Geometry check sheet. Reference: the model listing, model coordinates, mm. A direction names the side the tool comes from. Round coordinates to 2 decimals unless told otherwise and drop trailing zeros. Loops run counter-clockwise (first coordinate to the right, second up) from the corner with the lowest first, then second, coordinate; pieces in that order, holes last. Notation, with made-up numbers: M 74.5,19 L 128.5,19 A28 cw 128.5,54 Z; hole C 67,-1.75 d1. An arc over 180 degrees is marked long. Answer in a Markdown table with one row per item. Add a question column.
```python
from build123d import *

# Parameters (mm, degrees)
BOX_W           = 34.5
BOX_H           = 16
BOX_DEPTH       = 59
SKETCH_R        = 4
POCKET_DEPTH    = 34.501
POCKET001_DEPTH = 3.5000000001
BOX001_W        = 45
BOX001_H        = 9.5
BOX001_DEPTH    = 50
SKETCH008_R     = 1.75
POCKET002_DEPTH = 9.5010000001
PAD_DEPTH       = 8
PAD001_DEPTH    = 2
SKETCH009_R     = 3.5
POCKET003_DEPTH = 2
PAD002_DEPTH    = 50
SKETCH013_R     = 6
PAD003_DEPTH    = 17
SKETCH019_W     = 9
SKETCH019_H     = 5.5
PAD004_DEPTH    = 2
SKETCH015_W     = 3
SKETCH015_H     = 4
GROOVE_ANGLE    = 40
SKETCH016_W     = 3
SKETCH016_H     = 4
POCKET004_DEPTH = 5
SKETCH020_W     = 6.4
SKETCH020_H     = 3
PAD005_DEPTH    = 8
SKETCH021_R     = 1.7
POCKET005_DEPTH = 13
POCKET006_DEPTH = 15
SKETCH023_W     = 34.5
SKETCH023_H     = 2
POCKET007_DEPTH = 100


with BuildPart() as pocket001:
    # Box → Box (new body)
    with BuildSketch(Plane(origin=(-18, -8, -30), x_dir=(1, 0, 0), z_dir=(0, 0, 1))):
        with Locations((17.25, 8)):
            Rectangle(BOX_W, BOX_H)
    extrude(amount=BOX_DEPTH)

    # Sketch → Pocket (cut, through all)
    with BuildSketch(Plane(origin=(16.5, -8, -30), x_dir=(0, 1, 0), z_dir=(1, 0, 0))):
        with Locations((8, 51)):
            Circle(SKETCH_R)
        with Locations((8, 6)):
            Circle(SKETCH_R)
        with BuildLine():
            ThreePointArc((12.5, 39.4999793754), (8.0000103123, 44), (3.5, 39.5))
            Line((3.5, 39.5), (3.5, 14.5))
            Line((3.5, 14.5), (6, 12))
            Line((6, 12), (10, 12))
            Line((10, 12), (12.5, 14.5))
            Line((12.5, 14.5), (12.5, 39.4999793754))
        make_face()
    extrude(amount=-POCKET_DEPTH, mode=Mode.SUBTRACT)

    # Sketch007 → Pocket001 (cut)
    with BuildSketch(Plane(origin=(-18, 8, -30), x_dir=(-1, 0, 0), z_dir=(0, 1, 0))):
        Polygon((-34.5, 39.4999793754), (-24.8503628945, 27.9999896877), (-24.8503628945, 25.9999896877), (-34.5, 14.5), align=None)
    extrude(amount=-POCKET001_DEPTH, mode=Mode.SUBTRACT)


with BuildPart() as pocket007:
    # Box001 → Box001 (new body)
    with BuildSketch(Plane(origin=(16, -14, -30), x_dir=(1, 0, 0), z_dir=(0, 0, 1))):
        with Locations((22.5, 4.75)):
            Rectangle(BOX001_W, BOX001_H)
    extrude(amount=BOX001_DEPTH)

    # Sketch008 → Pocket002 (cut, through all)
    with BuildSketch(Plane(origin=(16, -14, -30), x_dir=(1, 0, 0), z_dir=(0, -1, 0))):
        with Locations((7, 44.5)):
            Circle(SKETCH008_R)
        with Locations((7, 13.5)):
            Circle(SKETCH008_R)
        with Locations((38, 13.5)):
            Circle(SKETCH008_R)
        Polygon((14, 50), (14, 43), (8.5, 37.5), (8.5, 21.5), (14, 16), (32.692131, 16), (32.692131, 18), (45, 18), (45, 50), align=None)
        Polygon((45, 9.1923881554), (35.8076118446, 0), (45, 0), align=None)
    extrude(amount=-POCKET002_DEPTH, mode=Mode.SUBTRACT)

    # Fusion: union Pocket001
    add(pocket001.part)

    # Sketch010 → Pad (new body)
    with BuildSketch(Plane(origin=(0, 0, -30), x_dir=(1, 0, 0), z_dir=(0, 0, -1))):
        with BuildLine():
            ThreePointArc((25.4999662688, 4.4999999999), (19.1360389694, 1.8639610307), (16.5000000001, -4.4999662687))
            Line((16.5000000001, -4.4999662687), (16.5000000001, 4.4999999999))
            Line((16.5000000001, 4.4999999999), (25.4999662688, 4.4999999999))
        make_face()
    extrude(amount=-PAD_DEPTH)

    # Sketch011 → Pad001 (new body)
    with BuildSketch(Plane.YZ.offset(16.5)):
        with BuildLine():
            ThreePointArc((-3.4641016151, -22), (0, -28), (3.4641016151, -22))
            Line((-3.4641016151, -22), (3.4641016151, -22))
        make_face()
    extrude(amount=-PAD001_DEPTH)

    # Sketch009 → Pocket003 (cut)
    with BuildSketch(Plane(origin=(0, -4.5, 0), x_dir=(-1, 0, 0), z_dir=(0, 1, 0))):
        with Locations((-23, 14.5)):
            Circle(SKETCH009_R)
        with Locations((-54, -16.5)):
            Circle(SKETCH009_R)
        with Locations((-23, -16.5)):
            Circle(SKETCH009_R)
    extrude(amount=-POCKET003_DEPTH, mode=Mode.SUBTRACT)

    # Sketch012 → Pad002 (new body)
    with BuildSketch(Plane(origin=(0, 0, -30), x_dir=(1, 0, 0), z_dir=(0, 0, -1))):
        with BuildLine():
            ThreePointArc((15.9999999999, 18.0000351724), (15.4138656704, 20.9466786767), (13.7447222151, 23.4447222151))
            Line((13.7447222151, 23.4447222151), (12.6133513652, 22.3133513652))
            ThreePointArc((11.6013945082, 23.1294048681), (4.4708258711, 13.2515870556), (12.6133513652, 22.3133513652))
            Line((11.6013945082, 23.1294048681), (12.4673340514, 24.4748225384))
            ThreePointArc((12.4673340514, 24.4748225384), (4.6120940547, 24.759389746), (0.6000000001, 18.0000351024))
            Line((0.6000000001, 18.0000351024), (0.6000000001, 8))
            Line((0.6000000001, 8), (15.9999999999, 8))
            Line((15.9999999999, 18.0000351724), (15.9999999999, 8))
        make_face()
    extrude(amount=-PAD002_DEPTH)

    # Sketch013 → Pad003 (new body)
    with BuildSketch(Plane(origin=(0, 0, -30), x_dir=(1, 0, 0), z_dir=(0, 0, -1))):
        with BuildLine():
            ThreePointArc((1.3480393737, 25.435516441), (-17.5103595019, 26.8672185857), (-16.2, 8))
            Line((-16.2, 8), (0.6000000001, 8))
            Line((0.6000000001, 8), (0.6, 18.0000060082))
            ThreePointArc((4.5689954494, 24.7356963295), (1.6660458786, 21.9090475457), (0.6, 18.0000060082))
            ThreePointArc((1.3480393737, 25.435516441), (2.8268537634, 24.4796180457), (4.5689954493, 24.7356963295))
        make_face()
        with Locations((-8.7, 18)):
            Circle(SKETCH013_R, mode=Mode.SUBTRACT)
    extrude(amount=-PAD003_DEPTH)

    # Sketch019 → Pad004 (new body)
    with BuildSketch(Plane.YZ.offset(16.5)):
        with Locations((0, 19.25)):
            Rectangle(SKETCH019_W, SKETCH019_H)
    extrude(amount=-PAD004_DEPTH)

    # Sketch015 → Groove (revolve, cut)
    with BuildSketch(Plane.XZ.offset(14)):
        with Locations((17.5, 5.5)):
            Rectangle(SKETCH015_W, SKETCH015_H)
    revolve(axis=Axis((0, -14, 0), (0, 0, 1)), revolution_arc=GROOVE_ANGLE, mode=Mode.SUBTRACT)

    # Sketch016 → Pocket004 (cut)
    with BuildSketch(Plane.XZ.offset(8)):
        with Locations((-0.8999999999, 5.5)):
            Rectangle(SKETCH016_W, SKETCH016_H)
    extrude(amount=-POCKET004_DEPTH, mode=Mode.SUBTRACT)

    # Sketch020 → Pad005 (new body)
    with BuildSketch(Plane(origin=(0, 0, -30), x_dir=(1, 0, 0), z_dir=(0, 0, -1))):
        Polygon((-19.3039162536, 24.6186826549), (-12.2, 36), (-5.2, 36), (1.3480393737, 25.435516441), align=None)
        with Locations((-8.7, 32)):
            Rectangle(SKETCH020_W, SKETCH020_H, mode=Mode.SUBTRACT)
    extrude(amount=-PAD005_DEPTH)

    # Sketch021 → Pocket005 (cut)
    with BuildSketch(Plane.XZ.offset(36)):
        with Locations((-8.7, -26)):
            Circle(SKETCH021_R)
    extrude(amount=-POCKET005_DEPTH, mode=Mode.SUBTRACT)

    # Sketch022 → Pocket006 (cut, symmetric)
    with BuildSketch(Plane.XY.offset(-13)):
        Polygon((-3.7636551984, -26.55), (1.1726896031, -18), (-3.7636551984, -9.45), (-13.6363448016, -9.45), (-18.5726896031, -18), (-13.6363448016, -26.55), align=None)
    extrude(amount=POCKET006_DEPTH, both=True, mode=Mode.SUBTRACT)

    # Sketch023 → Pocket007 (cut)
    with BuildSketch(Plane.XY.offset(29)):
        with Locations((-0.75, 7)):
            Rectangle(SKETCH023_W, SKETCH023_H)
    extrude(amount=-POCKET007_DEPTH, mode=Mode.SUBTRACT)


solid = pocket007.part
```
1) Go/stop test with flat-tipped pins: pin 1 (5 mm diameter, centred on x = 15, y = -9, fed in from +Z); pin 2 (15.5 mm diameter, centred on x = -8.7, y = -18, fed in from +Z); pin 3 (1 mm diameter, centred on y = -6, z = 5.5, fed in from +X); pin 4 (10.5 mm diameter, centred on y = -9.5, z = 3.5, fed in from +X). Record where each tip stops, or that it passes through.
2) Draft check along Y on faces 5 (the cylindrical face through (-0.509, -0.521, -20.034)), 6 (the flat face through (39, -9, -14)), 7 (the flat face through (33, -14, -16)). Enter one of: +Y half, -Y half, draft (parallel to the pull), parting line (faces both ways), or undercut.
3) Cross-section at B-B, the plane x = 23. Record the boundary of the cut face in (y, z), plus the area to 3 significant figures.
4) Cross-section at D-D, the plane x = 54. Record the boundary of the cut face in (y, z), plus the area to 3 significant figures.
5) Cross-section at C-C, the plane z = 21. Record the boundary of the cut face in (x, y).
6) Thickness scan on L1, parallel to Z at x = 23, y = -5.75; L2, parallel to Y at x = 8.3, z = 3.5; L3, parallel to Y at x = -8, z = -2. Record the ranges inside material, lowest first. Write a range as [from, to].
7) Cross-section at A-A, the plane y = -13. Count the separate pieces of the cut face and the enclosed holes in it, plus the area to 3 significant figures.
8) Set-up check for faces 1 (the flat face through (-9, -9.45, -20)), 2 (the flat face through (48.692, -9, -13)), 3 (the flat face through (55, -9, -12)), 4 (the flat face through (-18, -6, -1)): record each of +Z, -Z, +X, -X, +Y, -Y from which the full face is reachable in a straight line by a thin tool's end or side.
Worked answers:
| question | item | result |
|---|---|---|
| 1 | pin 1 | stops at z = 29 |
| 1 | pin 2 | stops at z = -28 |
| 1 | pin 3 | stops at x = 24.5 |
| 1 | pin 4 | stops at x = 25.75 |
| 2 | face 5 | undercut |
| 2 | face 6 | draft |
| 2 | face 7 | -Y half |
| 3 | outline | M -14,-30 L -4.15,-30 L -4.15,-22 L -4.5,-22 L -4.5,-20 L -6.5,-20 L -6.5,-18.25 L -14,-18.25 Z; M -14,-14.75 L -6.5,-14.75 L -6.5,-13 L -4.5,-13 L -4.5,11 L -6.5,11 L -6.5,12.75 L -14,12.75 Z; M -14,16.25 L -6.5,16.25 L -6.5,18 L -4.5,18 L -4.5,20 L -14,20 Z |
| 3 | area | 397 mm2 |
| 4 | outline | M -14,-27.81 L -4.5,-27.81 L -4.5,-20 L -6.5,-20 L -6.5,-18.25 L -14,-18.25 Z; M -14,-14.75 L -6.5,-14.75 L -6.5,-13 L -4.5,-13 L -4.5,-12 L -14,-12 Z |
| 4 | area | 110 mm2 |
| 5 | outline | M -18,-8 L 16.5,-8 L 16.5,6 L -18,6 L -18,4 L 14.5,4 L 14.5,-4 L -18,-4 Z |
| 6 | L1 | z = [-30, -20], [-13, 11], [18, 20] |
| 6 | L2 | y = [-25.7, -24.1], [-11.9, -4.5], [4.5, 6] |
| 6 | L3 | y = [-8, -4.5], [4.5, 6] |
| 7 | separate pieces | 3 |
| 7 | enclosed holes | 4 |
| 7 | area | 1,570 mm2 |
| 8 | face 1 | +Z |
| 8 | face 2 | +Z, +Y, -Y |
| 8 | face 3 | +Z, +X, +Y, -Y |
| 8 | face 4 | +Z, -Z, -X, +Y |
